from build123d import *

# Parameters (mm, degrees)
F1_DEPTH = 95
F4_DEPTH = 25
F3_W     = 59
F3_H     = 19.5249739359
F5_DEPTH = 25


# Not quite as in the source:
# - a feature names something its author has since deleted; it is built from what else it names


with BuildPart() as f1:
    # F0 (on Right) → F1 (new body)
    with BuildSketch(Plane.YZ):
        Polygon((-37.6999974251, 2.400000114), (22.3000025749, 2.400000114), (22.3000025749, 58.400000114), (12.3000025749, 58.400000114), (12.3000025749, 30.400000114), (-37.6999974251, 15.400000114), align=None)
    extrude(amount=F1_DEPTH)

    # F2 (on face) → F4 (cut)
    with BuildSketch(Plane.XZ.offset(-12.3000025749)):
        Polygon((95, 58.400000114), (33.3666242659, 58.400000114), (95, 30.400000114), align=None)
    extrude(amount=-F4_DEPTH, mode=Mode.SUBTRACT)

    # F3 (on face) → F5 (cut)
    with BuildSketch(Plane(origin=(0, 0, 2.400000114), x_dir=(1, 0, 0), z_dir=(0, 0, -1))):
        with Locations((48.5, 27.9375104571)):
            Rectangle(F3_W, F3_H)
    extrude(amount=-F5_DEPTH, mode=Mode.SUBTRACT)


solid = f1.part
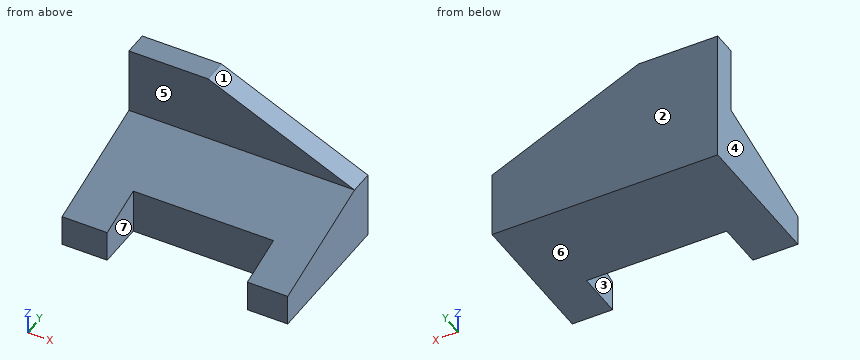
Here's how the part is built. I have some questions about the finished solid (model axes, mm). Face numbers are marked on the shaded views. A direction names the side the tool comes from. Coordinates: 2 decimals unless noted, no trailing zeros. Order: outer loops, then holes, each group sorted by start corner. A loop starts at its lowest first (then second) coordinate and runs counter-clockwise, first axis right, second up.
Item 1: If we section it at B-B on x = 9: List the corners of the cut face in (y, z) for me, plus the area to 4 significant figures.
Result sheet:
outline: (-37.7, 2.4) - (22.3, 2.4) - (22.3, 58.4) - (12.3, 58.4) - (12.3, 30.4) - (-37.7, 15.4) - close
area: 1,585 mm2
Item 2: For the marked faces 5, 6 and 7, which set-ups out of +Z, -Z, +X, -X, +Y, -Y let a thin tool reach every point of the face, with its end or its side?
Result sheet:
face 5: +Z, +X, -X, -Y
face 6: -Z, +X, -X, +Y, -Y
face 7: +Z, -Z, -Y
Item 3: If we mould it in two halves opening along X, with no side actions, what happens to the marked faces 1, 2, 3 and 4? For each: +X half, -X half, draft (parallel to the pull), parting line (faces both ways), or undercut.
Result sheet:
face 1: +X half
face 2: draft
face 3: undercut
face 4: -X half
Item 4: If we section it at C-C on y = -23: List the corners of the cut face in (x, z) for me.
Result sheet:
outline: (0, 2.4) - (19, 2.4) - (19, 19.81) - (0, 19.81) - close; (78, 2.4) - (95, 2.4) - (95, 19.81) - (78, 19.81) - close
Item 5: If we section it at A-A on y = -34: List the corners of the cut face in (x, z) for me.
Result sheet:
outline: (0, 2.4) - (19, 2.4) - (19, 16.51) - (0, 16.51) - close; (78, 2.4) - (95, 2.4) - (95, 16.51) - (78, 16.51) - close
Item 6: I need wall thicknesses on line 1 (X direction, y = -30, z = 16.5); line 2 (Y direction, x = 47.5, z = 38.5); line 3 (Y direction, x = 59.5, z = 9). Which ranges of each line are inside material? Lowest first, please.
Result sheet:
line 1: x = 0 to 19, 78 to 95
line 2: y = 12.3 to 22.3
line 3: y = -18.18 to 22.3
Item 7: If we section it at D-D on z = 25: List the corners of the cut face in (x, y) for me.
Result sheet:
outline: (0, -5.7) - (95, -5.7) - (95, 22.3) - (0, 22.3) - close
Item 8: For P1, Ø1.5, axis at x = 48.5, y = -15, coming from the +Z side (3 decimals); P2, Ø5, axis at x = 44, y = -0.5, coming from the +Z side; P3, Ø5, axis at x = 16, z = 42, coming from the -Y side, each with a flat end and sliding along its axis, tell me the tip position at first contact or that it passes through.
Result sheet:
P1: stops at z = 22.435
P2: stops at z = 27.31
P3: stops at y = 12.3
